from build123d import *

# Parameters (mm, degrees)
BASPROSKE_W        = 10
BASPROSKE_H        = 15.75
TOOTHCUT_DEPTH     = 25.415671197
TEETHCUTS_COUNT    = 26
TEETHCUTS_ANGLE    = 346.153846154
BORSKE_R           = 4
BORE_DEPTH         = 50.0000508
SKETCH1_R          = 2
CUT_EXTRUDE2_DEPTH = 5
SKETCH2_R          = 1
CUT_EXTRUDE3_DEPTH = 10


with BuildPart() as part:
    # BasProSke → Base-Revolve (revolve)
    with BuildSketch(Plane(origin=(0, 0, 0), x_dir=(1, 0, 0), z_dir=(0, 1, 0)), mode=Mode.PRIVATE) as base_revolve_sk:
        with Locations((5, 7.875)):
            Rectangle(BASPROSKE_W, BASPROSKE_H)
    revolve(base_revolve_sk.sketch.rotate(Axis((-10, 0, 0), (1, 0, 0)), 180), axis=Axis((-10, 0, 0), (1, 0, 0)))

    # TooCutSke → ToothCut (cut, through all)
    with BuildSketch(Plane(origin=(0, 0, 0), x_dir=(0, 0, -1), z_dir=(1, 0, 0))):
        with BuildLine():
            ThreePointArc((0.637727704, 13.202356549), (0, 13.21775), (-0.637727704, 13.202356549))
            ThreePointArc((-0.637727704, 13.202356549), (-0.924330219, 14.50249659), (-1.497477225, 15.704165279))
            ThreePointArc((-1.497477225, 15.704165279), (0, 15.7754), (1.497477225, 15.704165279))
            ThreePointArc((1.497477225, 15.704165279), (0.924330219, 14.50249659), (0.637727704, 13.202356549))
        make_face()
    toothcut = extrude(amount=TOOTHCUT_DEPTH, mode=Mode.SUBTRACT)

    # TeethCuts: ToothCut ×26 about axis
    teethcuts_axis = Axis((-10, 0, 0), (1, 0, 0))
    for i in range(1, TEETHCUTS_COUNT):
        add(toothcut.rotate(teethcuts_axis, i * TEETHCUTS_ANGLE / (TEETHCUTS_COUNT - 1)), mode=Mode.SUBTRACT)

    # BorSke → Bore (cut, symmetric)
    with BuildSketch(Plane(origin=(0, 0, 0), x_dir=(0, 0, -1), z_dir=(1, 0, 0))):
        with Locations(Location((0, 0, 0), (0, 0, 180))):
            Circle(BORSKE_R)
    extrude(amount=BORE_DEPTH, both=True, mode=Mode.SUBTRACT)

    # Sketch1 → Cut-Extrude2 (cut)
    with BuildSketch(Plane(origin=(10, 0, 0), x_dir=(0, 0, -1), z_dir=(1, 0, 0))):
        with Locations((8, 0)):
            Circle(SKETCH1_R)
        with Locations((0, -8)):
            Circle(SKETCH1_R)
        with Locations((-8, 0)):
            Circle(SKETCH1_R)
        with Locations((0, 8)):
            Circle(SKETCH1_R)
    extrude(amount=-CUT_EXTRUDE2_DEPTH, mode=Mode.SUBTRACT)

    # Sketch2 → Cut-Extrude3 (cut)
    with BuildSketch(Plane(origin=(10, 0, 0), x_dir=(0, 0, -1), z_dir=(1, 0, 0))):
        with Locations((8, 0)):
            Circle(SKETCH2_R)
        with Locations((0, -8)):
            Circle(SKETCH2_R)
        with Locations((-8, 0)):
            Circle(SKETCH2_R)
        with Locations((0, 8)):
            Circle(SKETCH2_R)
    extrude(amount=-CUT_EXTRUDE3_DEPTH, mode=Mode.SUBTRACT)


solid = part.part
Verification items for the finished model (mm, model axes). A direction names the side the tool comes from. Give positions to 0.01 mm unless a question says otherwise; leave off trailing zeros. Write each loop counter-clockwise with the first axis right and the second up, starting at its lowest first coordinate (ties: lowest second). Pieces come first, ordered by that corner, then holes. Notation, with made-up numbers: M 4.25,3 L 56.25,3 A26 ccw 56.25,23 Z; hole C -34.5,82.25 d4. An arc over 180 degrees is marked long. Put each result on its own line as item: value. Start each with the question number.
1. Go/stop test with flat-tipped pins: pin 1 Ø4 at (x, y) = (7, 1) entering from +Z; pin 2 Ø4 at (x, y) = (5.5, 5.5) entering from -Z; pin 3 Ø1.6 at (y, z) = (-8, 0) entering from +X; pin 4 Ø1.2 at (y, z) = (0.5, 8.5) entering from +X. Record where each tip stops, or that it passes through.
2. Scan lines: line 1 along Y through (x, z) = (6.5, 0); line 2 along Y through (x, z) = (4.25, -8.5); line 3 along Y through (x, z) = (4.75, 14). Record each from-to range of solid material in increasing order. Write a range as [from, to].
3. Section check B-B (y = 0). Record the cut outline in (x, z).
4. Set-up check for faces 1 (the face through (4.93, -2.651, 14.256)), 2 (the face through (5, 7, -1)), 3 (the face through (4.93, 13.86, -4.37)), 4 (the face through (4.93, 2.651, -14.256)), 5 (the face through (4.93, -14.307, -2.573)): record each of +Z, -Z, +X, -X, +Y, -Y from which the full face is reachable in a straight line by a thin tool's end or side.
5. Section check C-C (x = 8). Give the number of separate pieces and of enclosed holes in the cut face, and give its area (3 significant figures).
6. Section check A-A (z = 0). Record the cut outline in (x, y).
Answer list:
1. pin 1: z = 15.75
1. pin 2: z = -15.36
1. pin 3: through
1. pin 4: x = 5
2. line 1: [-13.22, -10], [-6, -4], [4, 6], [10, 13.22]
2. line 2: [-13.13, -10.64], [-10.12, -0.87], [0.87, 10.12], [10.64, 13.13]
2. line 3: [-7.22, -6.78], [-4.28, -2.54], [-0.92, 0.92], [2.54, 4.28], [6.78, 7.22]
3. outline: M 0,-15.75 L 10,-15.75 L 10,-10 L 5,-10 L 5,-9 L 0,-9 Z; M 0,-7 L 5,-7 L 5,-6 L 10,-6 L 10,-4 L 0,-4 Z; M 0,4 L 10,4 L 10,6 L 5,6 L 5,7 L 0,7 Z; M 0,9 L 5,9 L 5,10 L 10,10 L 10,15.75 L 0,15.75 Z
4. face 1: +Z, +X, -X
4. face 2: +X
4. face 3: +X, -X, +Y
4. face 4: -Z, +X, -X
4. face 5: +X, -X
5. separate pieces: 1
5. enclosed holes: 5
5. area: 552 mm2
6. outline: M 0,-13.22 L 10,-13.22 L 10,-10 L 5,-10 L 5,-9 L 0,-9 Z; M 0,-7 L 5,-7 L 5,-6 L 10,-6 L 10,-4 L 0,-4 Z; M 0,4 L 10,4 L 10,6 L 5,6 L 5,7 L 0,7 Z; M 0,9 L 5,9 L 5,10 L 10,10 L 10,13.22 L 0,13.22 Z
